from build123d import *

# Parameters (mm, degrees)
SKETCH1_W               = 104
SKETCH1_H               = 92
BOSS_EXTRUDE1_DEPTH     = 38
SHELL1_T                = 6
SKETCH15_W              = 3
SKETCH15_H              = 44
CUT_EXTRUDE4_DEPTH      = 133.680066325
SKETCH3_W               = 8
SKETCH3_H               = 12
SKETCH3_W_2             = 18
SKETCH3_H_2             = 7
SKETCH3_W_3             = 16
SKETCH3_H_3             = 14
SKETCH3_W_4             = 31
SKETCH3_H_4             = 17
SKETCH3_W_5             = 10
SKETCH3_H_5             = 4
CUT_EXTRUDE2_DEPTH      = 10
CUT_EXTRUDE5_DEPTH      = 118.613774703
CUT_EXTRUDE5_DEPTH_BACK = 118.613774703
SKETCH3_3_W             = 5.5
SKETCH3_3_H             = 44
CUT_EXTRUDE3_DEPTH      = 122.512345052
CUT_EXTRUDE3_DEPTH_BACK = 122.512345052
BOSS_EXTRUDE2_DEPTH     = 3
BOSS_EXTRUDE3_START     = -3
BOSS_EXTRUDE3_OUTLINE_W = 105
BOSS_EXTRUDE3_OUTLINE_H = 3
BOSS_EXTRUDE3_DEPTH     = 3
BOSS_EXTRUDE4_START     = -3
BOSS_EXTRUDE4_OUTLINE_W = 105
BOSS_EXTRUDE4_OUTLINE_H = 3
BOSS_EXTRUDE4_DEPTH     = 3


# Read off the part's stored shape, not the designer's step: Boss-Extrude3, Boss-Extrude4
with BuildPart() as part:
    # Sketch1 → Boss-Extrude1 (new body)
    with BuildSketch(Plane(origin=(0, 0, 0), x_dir=(1, 0, 0), z_dir=(0, 1, 0))):
        Rectangle(SKETCH1_W, SKETCH1_H)
    extrude(amount=BOSS_EXTRUDE1_DEPTH)

    # Shell1
    shell1_openings = [part.faces().sort_by_distance(p)[0] for p in [
        (0, 38, 0),
    ]]
    offset(amount=SHELL1_T, openings=shell1_openings, kind=Kind.INTERSECTION)

    # Sketch15 → Cut-Extrude4 (cut, through all)
    with BuildSketch(Plane(origin=(58, 0, 0), x_dir=(0, 0, -1), z_dir=(1, 0, 0))):
        with Locations((-50.5, 16)):
            Rectangle(SKETCH15_W, SKETCH15_H)
        with Locations((50.5, 16)):
            Rectangle(SKETCH15_W, SKETCH15_H)
    extrude(amount=-CUT_EXTRUDE4_DEPTH, mode=Mode.SUBTRACT)

    # Sketch3 → Cut-Extrude2 (cut)
    with BuildSketch(Plane(origin=(0, 0, 46), x_dir=(-1, 0, 0), z_dir=(0, 0, -1))):
        with Locations((41.5, 11)):
            Rectangle(SKETCH3_W, SKETCH3_H)
        with Locations((25.5, 8.5)):
            Rectangle(SKETCH3_W_2, SKETCH3_H_2)
        with Locations((-27.5, 12)):
            Rectangle(SKETCH3_W_3, SKETCH3_H_3)
        with Locations((-2, 13.5)):
            Rectangle(SKETCH3_W_4, SKETCH3_H_4)
        with Locations((-42.5, 7)):
            Rectangle(SKETCH3_W_5, SKETCH3_H_5)
    extrude(amount=-CUT_EXTRUDE2_DEPTH, mode=Mode.SUBTRACT)

    # Sketch3<3> → Cut-Extrude5 (cut, two sides: drawn at the far end of the back side and taken through both)
    with BuildSketch(Plane(origin=(0, 0, 46), x_dir=(-1, 0, 0), z_dir=(0, 0, -1)).offset(-CUT_EXTRUDE5_DEPTH_BACK)):
        with Locations((55.25, 16)):
            Rectangle(SKETCH3_3_W, SKETCH3_3_H)
        with Locations((-55.25, 16)):
            Rectangle(SKETCH3_3_W, SKETCH3_3_H)
    extrude(amount=CUT_EXTRUDE5_DEPTH + CUT_EXTRUDE5_DEPTH_BACK, mode=Mode.SUBTRACT)

    # Sketch4 → Cut-Extrude3 (cut, two sides: drawn at the far end of the back side and taken through both)
    with BuildSketch(Plane(origin=(-52, 0, 0), x_dir=(0, 0, -1), z_dir=(1, 0, 0)).offset(-CUT_EXTRUDE3_DEPTH_BACK)):
        Polygon((-46, 257.389589044), (-46, 38), (-46, 0), (46, 0), (46, 38), (46, 257.389589044), (46, 696.168767132), (-46, 696.168767132), align=None)
    extrude(amount=CUT_EXTRUDE3_DEPTH + CUT_EXTRUDE3_DEPTH_BACK, mode=Mode.SUBTRACT)

    # Sketch10 → Boss-Extrude2 (add)
    with BuildSketch(Plane(origin=(0, 0, 46), x_dir=(-1, 0, 0), z_dir=(0, 0, -1))):
        Polygon((-37.576697733, 38), (-30.392876327, 38), (-31.48478703, 41), (-36.48478703, 41), align=None)
        Polygon((31.48478703, 41), (30.392876327, 38), (37.576697733, 38), (36.48478703, 41), align=None)
    boss_extrude2 = extrude(amount=-BOSS_EXTRUDE2_DEPTH)

    # Mirror3: Boss-Extrude2 across plane
    add(boss_extrude2.mirror(Plane.XY))

    # Boss-Extrude3 outline → Boss-Extrude3 (add)
    with BuildSketch(Plane(origin=(0, 0, -46), x_dir=(-1, 0, 0), z_dir=(0, 0, -1)).offset(BOSS_EXTRUDE3_START)):
        with Locations((0, 9)):
            Rectangle(BOSS_EXTRUDE3_OUTLINE_W, BOSS_EXTRUDE3_OUTLINE_H)
    extrude(amount=BOSS_EXTRUDE3_DEPTH)

    # Boss-Extrude4 outline → Boss-Extrude4 (add)
    with BuildSketch(Plane.XY.offset(46).offset(BOSS_EXTRUDE4_START)):
        with Locations((0, 24)):
            Rectangle(BOSS_EXTRUDE4_OUTLINE_W, BOSS_EXTRUDE4_OUTLINE_H)
    extrude(amount=BOSS_EXTRUDE4_DEPTH)

    # Sketch19 → CSK for #1 Flat Head Socket Cap Screw2 (revolve, cut)
    with BuildSketch(Plane(origin=(52.5, -3, 43.94), x_dir=(0, 0, -1), z_dir=(0, 1, 0))):
        Polygon((0, 0), (0, 35.618105319), (1.0287, 35), (1.0287, 1.271042053), (2.1336, 0), align=None)
    csk_for_1_flat_head_socket_cap_screw2 = revolve(axis=Axis((58.85, -3, 43.94), (-1, 0, 0)), mode=Mode.SUBTRACT)

    # Mirror4: CSK for #1 Flat Head Socket Cap Screw2 across plane
    add(csk_for_1_flat_head_socket_cap_screw2.mirror(Plane(origin=(0, 0, 0), x_dir=(0, 0, 1), z_dir=(1, 0, 0))), mode=Mode.SUBTRACT)

    # Mirror4 at the second plane: CSK for #1 Flat Head Socket Cap Screw2 across plane
    add(csk_for_1_flat_head_socket_cap_screw2.mirror(Plane.XY), mode=Mode.SUBTRACT)

    # Mirror4 at the second plane copy 1 sketc → Mirror4 at the second plane copy 1 (revolve, cut)
    with BuildSketch(Plane(origin=(-52.5, -3, -43.94), x_dir=(0, 0, 1), z_dir=(0, 1, 0))):
        Polygon((0, 0), (0, 35.618105319), (1.0287, 35), (1.0287, 1.271042053), (2.1336, 0), align=None)
    revolve(axis=Axis((-58.85, -3, -43.94), (1, 0, 0)), mode=Mode.SUBTRACT)


solid = part.part
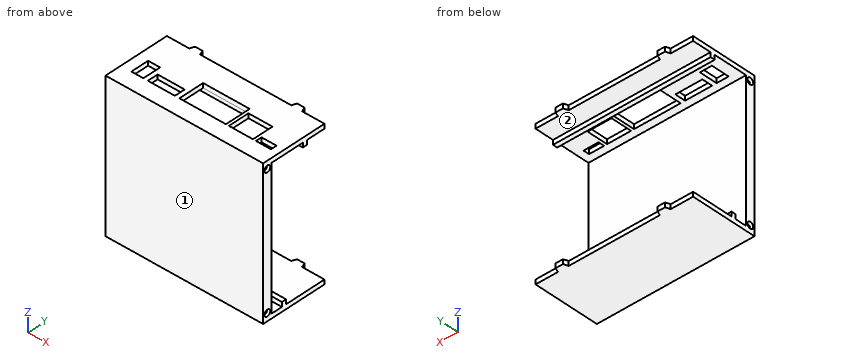
Verification items for the finished model (mm, model axes). Face numbers are marked on the shaded views. A direction names the side the tool comes from. Give positions to 0.01 mm unless a question says otherwise; leave off trailing zeros. Write each loop counter-clockwise with the first axis right and the second up, starting at its lowest first coordinate (ties: lowest second). Pieces come first, ordered by that corner, then holes. Notation, with made-up numbers: M -40,-0.5 L -13,-0.5 A18 ccw -13,17.5 Z; hole C -8.5,7 d10. An arc over 180 degrees is marked long. Put each result on its own line as item: value. Start each with the question number.
1. Section check D-D (x = -21). Record the cut outline in (y, z).
2. Section check A-A (x = 39). Record the cut outline in (y, z).
3. Section check C-C (y = 14.5). Record the cut outline in (x, z).
4. Section check B-B (x = -7.5). Record the cut outline in (y, z).
5. Set-up check for the marked faces 1 and 2: record each of +Z, -Z, +X, -X, +Y, -Y from which the full face is reachable in a straight line by a thin tool's end or side.
6. Go/stop test with flat-tipped pins: pin 1 Ø0.9 at (x, y) = (-12.5, 8.5) entering from +Z; pin 2 Ø0.9 at (x, z) = (-41.5, 48) entering from +Y; pin 3 Ø10 at (x, z) = (14.5, -24) entering from +Y. Record where each tip stops, or that it passes through.
7. Scan lines: line 1 along Z through (x, y) = (39.5, -3); line 2 along Y through (x, z) = (-40.5, 43.94); line 3 along Z through (x, y) = (23.5, 28). Record each from-to range of solid material in increasing order. Write a range as [from, to].
Answer list:
1. outline: M -6,-49 L 38,-49 L 38,-46 L 10.5,-46 L 10.5,-43 L 7.5,-43 L 7.5,-46 L 0,-46 L 0,46 L 5,46 L 5,49 L -6,49 Z; M 12,46 L 22.5,46 L 22.5,43 L 25.5,43 L 25.5,46 L 38,46 L 38,49 L 12,49 Z; hole C -3,-43.94 d2.06; hole C -3,43.94 d2.06
2. outline: M -6,-49 L 38,-49 L 38,-46 L 10.5,-46 L 10.5,-43 L 7.5,-43 L 7.5,-46 L 0,-46 L 0,46 L 5,46 L 5,49 L -6,49 Z; M 9,46 L 22.5,46 L 22.5,43 L 25.5,43 L 25.5,46 L 38,46 L 38,49 L 9,49 Z; hole C -3,-43.94 d2.06; hole C -3,43.94 d2.06
3. outline: M -52.5,-49 L 52.5,-49 L 52.5,-46 L -52.5,-46 Z; M -52.5,46 L -45.5,46 L -45.5,49 L -52.5,49 Z; M -37.5,46 L -13.5,46 L -13.5,49 L -37.5,49 Z; M 17.5,46 L 19.5,46 L 19.5,49 L 17.5,49 Z; M 35.5,46 L 52.5,46 L 52.5,49 L 35.5,49 Z
4. outline: M -6,-49 L 38,-49 L 38,-46 L 10.5,-46 L 10.5,-43 L 7.5,-43 L 7.5,-46 L 0,-46 L 0,46 L 5,46 L 5,49 L -6,49 Z; M 22,46 L 22.5,46 L 22.5,43 L 25.5,43 L 25.5,46 L 38,46 L 38,49 L 22,49 Z
5. face 1: +Z, -Z, +X, -X, -Y
5. face 2: +X, -X, +Y
6. pin 1: z = -43
6. pin 2: y = 38
6. pin 3: y = 0
7. line 1: [-49, -44.97], [-42.91, 42.91], [44.97, 49]
7. line 2: [-6, -4.03], [-1.97, 0], [22.5, 25.5]
7. line 3: [-49, -46], [46, 49]
